The drawing under review shows one solid part. Ordinate dimensions are in mm from its lowest x, y, z. A direction names the side the tool comes from. Coordinates: 2 decimals unless noted, no trailing zeros. Order: outer loops, then holes, each group sorted by start corner. A loop starts at its lowest first (then second) coordinate and runs counter-clockwise, first axis right, second up.
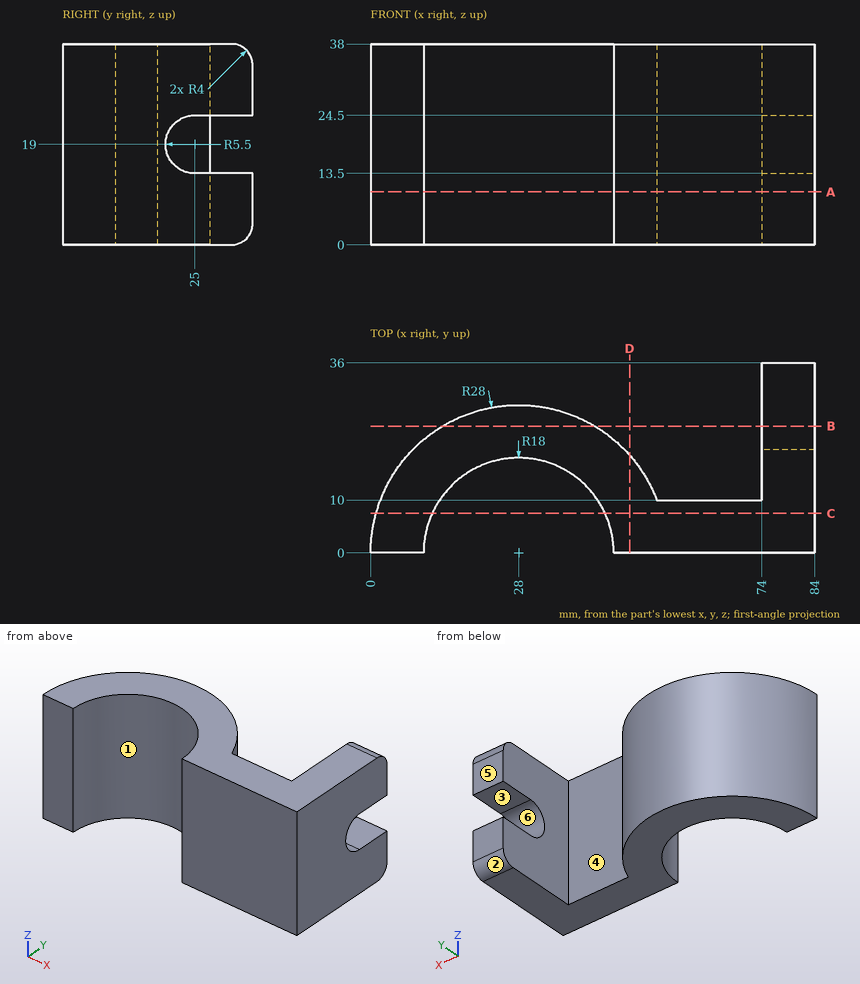
1. Take a section at C-C, the plane y = 7.5. Give the boundary of the cut face in (x, z), plus the area to 3 significant figures.
Answer below:
outline: (1.02, 0) - (11.64, 0) - (11.64, 38) - (1.02, 38) - close; (44.36, 0) - (84, 0) - (84, 38) - (44.36, 38) - close
area: 1,910 mm2
2. Clearance check with flat-ended pins moving along their axes: pin 1 Ø5 at (x, y) = (81, 28.5) entering from -Z; pin 2 Ø10 at (x, z) = (42, 31.5) entering from +Y; pin 3 Ø5 at (y, z) = (21, 21.5) entering from -X; pin 4 Ø10 at (x, z) = (20.5, 28.5) entering from +Y. State where each tip first meets the part, or that it passes through.
Answer below:
pin 1: stops at z = 0
pin 2: stops at y = 26.51
pin 3: stops at x = 6.98
pin 4: stops at y = 27.89
3. Take a section at B-B, the plane y = 24. Give the boundary of the cut face in (x, z).
Answer below:
outline: (13.58, 0) - (42.42, 0) - (42.42, 38) - (13.58, 38) - close; (74, 0) - (84, 0) - (84, 13.59) - (74, 13.59) - close; (74, 24.41) - (84, 24.41) - (84, 38) - (74, 38) - close
4. The part is to be moulded in two halves that separate along Z. For the marked faces 1, 2 and 3, say which applies: +Z half, -Z half, draft (parallel to the pull), parting line (faces both ways), or undercut.
Answer below:
face 1: draft
face 2: -Z half
face 3: undercut
5. To check wall thickness, follow L1, parallel to X at y = 16, z = 13; L2, parallel to X at y = 13, z = 16; L3, parallel to X at y = 24, z = 11. State the ranges of each line that lie inside material, in increasing order.
Answer below:
L1: x = 5.02 to 19.75, 36.25 to 50.98, 74 to 84
L2: x = 3.2 to 15.55, 40.45 to 52.8, 74 to 84
L3: x = 13.58 to 42.42, 74 to 84
6. Take a section at D-D, the plane x = 49. Give the boundary of the cut face in (y, z).
Answer below:
outline: (0, 0) - (18.52, 0) - (18.52, 38) - (0, 38) - close
7. Machinability: for the marked faces 4, 5 and 6, which of the approach directions +Z, -Z, +X, -X, +Y, -Y give a long, thin tool a straight path to every point of the face, cutting with its end or side? Answer none if there is none.
Answer below:
face 4: +Z, -Z, +Y
face 5: +Z, -Z, +X, -X, +Y
face 6: +X, +Y
8. Take a section at A-A, the plane z = 10. Give the boundary of the cut face in (x, y), plus the area to 3 significant figures.
Answer below:
outline: (0, 0) - (10, 0) arc R18 cw to (46, 0) - (84, 0) - (84, 36) - (74, 36) - (74, 10) - (54.15, 10) arc R28 ccw to start
area: 1,270 mm2
